from build123d import *

# Parameters (mm, degrees)
SKETCH1_R           = 1.8288
BOSS_EXTRUDE1_DEPTH = 3.175
SKETCH3_R           = 1.5
CUT_EXTRUDE1_DEPTH  = 4.175
SKETCH4_R           = 1.4732
CUT_EXTRUDE2_DEPTH  = 4.175
SKETCH5_R           = 1.524
SKETCH5_W           = 10.16
SKETCH5_H           = 3.81
CUT_EXTRUDE3_DEPTH  = 4.175


with BuildPart() as part:
    # Sketch1 → Boss-Extrude1 (new body)
    with BuildSketch(Plane(origin=(0, 0, 0), x_dir=(1, 0, 0), z_dir=(0, 1, 0))):
        Polygon((-226.6315, 82.55), (-194.8815, 82.55), (-194.8815, 69.85), (-188.5315, 69.85), (-188.5315, 82.55), (-38.1, 82.55), (-38.1, 69.85), (-31.75, 69.85), (-31.75, 82.55), (0, 82.55), (0, 51.435), (-3.175, 51.435), (-3.175, 31.115), (0, 31.115), (0, 0), (-31.75, 0), (-31.75, 12.7), (-38.1, 12.7), (-38.1, 0), (-188.5315, 0), (-188.5315, 12.7), (-194.8815, 12.7), (-194.8815, 0), (-226.6315, 0), (-226.6315, 31.115), (-223.4565, 31.115), (-223.4565, 51.435), (-226.6315, 51.435), align=None)
        with Locations((-113.31575, 41.275)):
            Circle(SKETCH1_R, mode=Mode.SUBTRACT)
    extrude(amount=BOSS_EXTRUDE1_DEPTH)

    # Sketch3 → Cut-Extrude1 (cut, through all)
    with BuildSketch(Plane(origin=(0, 3.175, 0), x_dir=(1, 0, 0), z_dir=(0, 1, 0))):
        with Locations((-106.7, 29.08)):
            Circle(SKETCH3_R)
        with Locations((-106.7, 5.08)):
            Circle(SKETCH3_R)
        with Locations((-12.7, 5.08)):
            Circle(SKETCH3_R)
        with Locations((-12.7, 29.08)):
            Circle(SKETCH3_R)
    extrude(amount=-CUT_EXTRUDE1_DEPTH, mode=Mode.SUBTRACT)

    # Sketch4 → Cut-Extrude2 (cut, through all)
    with BuildSketch(Plane(origin=(0, 3.175, 0), x_dir=(1, 0, 0), z_dir=(0, 1, 0))):
        with Locations((-150.4315, 49.53)):
            Circle(SKETCH4_R)
        with Locations((-150.4315, 74.93)):
            Circle(SKETCH4_R)
        with Locations((-201.2315, 74.93)):
            Circle(SKETCH4_R)
        with Locations((-201.2315, 49.53)):
            Circle(SKETCH4_R)
    extrude(amount=-CUT_EXTRUDE2_DEPTH, mode=Mode.SUBTRACT)

    # Sketch5 → Cut-Extrude3 (cut, through all)
    with BuildSketch(Plane(origin=(0, 3.175, 0), x_dir=(1, 0, 0), z_dir=(0, 1, 0))):
        with Locations((-203.369556456, 14.996771974)):
            Circle(SKETCH5_R)
        with Locations((-148.759556456, 14.996771974)):
            Circle(SKETCH5_R)
        with Locations((-25.4, 58.913810593)):
            Circle(SKETCH5_R)
        with Locations((-119.38, 58.913810593)):
            Circle(SKETCH5_R)
        with Locations((-177.797598384, 33.655)):
            Rectangle(SKETCH5_W, SKETCH5_H)
        with Locations((-66.164783375, 43.089749173)):
            Rectangle(SKETCH5_W, SKETCH5_H)
        with Locations((-66.164783375, 77.379749173)):
            Rectangle(SKETCH5_W, SKETCH5_H)
    extrude(amount=-CUT_EXTRUDE3_DEPTH, mode=Mode.SUBTRACT)


solid = part.part
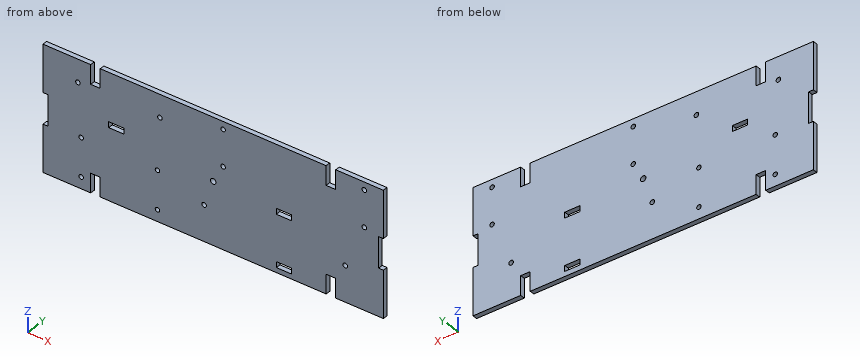
The listing builds one solid part. Answer for the finished solid, in the listing's coordinates (mm). Give positions to 0.01 mm unless a question says otherwise; leave off trailing zeros.
Item 1: Flat-ended cylindrical pins translate along their axes: P1, Ø1.6, axis at y = 1, z = -44, coming from the -X side; P2, Ø1, axis at x = -36, y = 1.5, coming from the -Z side. Find the tip coordinate at first contact, or state that the pin passes through.
Item 2: Section A-A, the plane y = 0.75 is taken. Count the separate pieces of the cut face and the enclosed holes in it, plus the area to 3 significant figures.
Item 3: Find the intervals of material crossed by line 1 along X through (y, z) = (1.8, -29.08); line 2 along X through (y, z) = (1.5, -74.93); line 3 along X through (y, z) = (1.75, -5.08), in increasing order.
Completed:
1. P1: stops at x = -223.46
1. P2: stops at z = -69.85
2. separate pieces: 1
2. enclosed holes: 16
2. area: 18,000 mm2
3. line 1: x = -226.63 to -108.2, -105.2 to -14.2, -11.2 to 0
3. line 2: x = -226.63 to -202.7, -199.76 to -194.88, -188.53 to -151.9, -148.96 to -38.1, -31.75 to 0
3. line 3: x = -226.63 to -194.88, -188.53 to -108.2, -105.2 to -38.1, -31.75 to -14.2, -11.2 to 0
